from build123d import *

# Parameters (mm, degrees)
SKETCH1_R           = 2.1
BOSS_EXTRUDE1_DEPTH = 3
EXTRUDE_THIN1_DEPTH = 47
BOSS_EXTRUDE2_DEPTH = 3
SKETCH4_W           = 31
SKETCH4_H           = 51
CUT_EXTRUDE1_DEPTH  = 72.0791812
FILLET3_R           = 5
BOSS_EXTRUDE3_DEPTH = 30
FILLET1_R           = 5
CUT_EXTRUDE3_REACH  = 75.33
SKETCH10_R          = 0.5
SKETCH11_R          = 4.15
CUT_EXTRUDE4_DEPTH  = 1
FILLET2_R           = 5


with BuildPart() as part:
    # Sketch1 → Boss-Extrude1 (new body)
    with BuildSketch(Plane.XY):
        with BuildLine():
            Line((7.416198487, 5), (23.5, 5))
            Line((23.5, 5), (23.5, -25))
            Line((23.5, -25), (-23.5, -25))
            Line((-23.5, -25), (-23.5, 5))
            Line((-23.5, 5), (-7.416198487, 5))
            ThreePointArc((-7.416198487, 5), (0, 0), (7.416198487, 5))
        make_face()
        with Locations((-17.5, 0)):
            Circle(SKETCH1_R, mode=Mode.SUBTRACT)
        with Locations(Location((17.5, 0, 0), (0, 0, 180))):
            Circle(SKETCH1_R, mode=Mode.SUBTRACT)
    extrude(amount=BOSS_EXTRUDE1_DEPTH)

    # Sketch2 → Extrude-Thin1 (add)
    with BuildSketch(Plane.ZY.offset(23.5)):
        Polygon((0, -25), (-60, -25), (-60, 5), (-57, 5), (-57, -22), (0, -22), align=None)
    extrude(amount=-EXTRUDE_THIN1_DEPTH)

    # Sketch3 → Boss-Extrude2 (add)
    with BuildSketch(Plane.ZY.offset(23.5)):
        Polygon((-57, 5), (-57, -22), (0, -22), (0, 5), (-17.944444444, -12), (-39.055555556, -12), align=None)
    boss_extrude2 = extrude(amount=-BOSS_EXTRUDE2_DEPTH)

    # Mirror1: Boss-Extrude2 across plane
    add(boss_extrude2.mirror(Plane(origin=(0, 0, 0), x_dir=(0, 0, 1), z_dir=(1, 0, 0))))

    # Sketch4 → Cut-Extrude1 (cut, through all)
    with BuildSketch(Plane.XZ.offset(25)):
        with Locations((0, -28.5)):
            Rectangle(SKETCH4_W, SKETCH4_H)
    extrude(amount=-CUT_EXTRUDE1_DEPTH, mode=Mode.SUBTRACT)

    # Fillet3
    fillet3_edges = [part.edges().sort_by_distance(p)[0] for p in [
        (15.5, -23.5, -3),
        (15.5, -23.5, -54),
        (-15.5, -23.5, -54),
        (-15.5, -23.5, -3),
    ]]
    fillet(fillet3_edges, radius=FILLET3_R)

    # Sketch6 → Boss-Extrude3 (add)
    with BuildSketch(Plane(origin=(0, 5, 0), x_dir=(1, 0, 0), z_dir=(0, 1, 0))):
        Polygon((20.5, 57), (23.5, 57), (23.5, 60), (-23.5, 60), (-23.5, 57), (-20.5, 57), align=None)
    extrude(amount=BOSS_EXTRUDE3_DEPTH)

    # Fillet1
    fillet1_edges = [part.edges().sort_by_distance(p)[0] for p in [
        (-20.5, -22, -28.5),
        (20.5, -22, -28.5),
    ]]
    fillet(fillet1_edges, radius=FILLET1_R - 0.0001)  # a hair under: the kernel refuses the full size

    # Sketch10 → Cut-Extrude3 (cut, up to next)
    with BuildSketch(Plane.XY.offset(-57), mode=Mode.PRIVATE) as cut_extrude3_sk1:
        with Locations((0, 8)):
            Circle(SKETCH10_R)
    cut_extrude3_tool1 = extrude(cut_extrude3_sk1.sketch, amount=-CUT_EXTRUDE3_REACH, mode=Mode.PRIVATE) & part.part
    add(cut_extrude3_tool1.solids().sort_by_distance((0, 8, -57))[0], mode=Mode.SUBTRACT)

    # Sketch11 → Cut-Extrude4 (cut)
    with BuildSketch(Plane(origin=(0, 0, -60), x_dir=(-1, 0, 0), z_dir=(0, 0, -1))):
        with Locations((-18.5, 30)):
            Circle(SKETCH11_R)
        with Locations((18.5, 30)):
            Circle(SKETCH11_R)
        with Locations((-18.5, -20)):
            Circle(SKETCH11_R)
        with Locations((18.5, -20)):
            Circle(SKETCH11_R)
    extrude(amount=-CUT_EXTRUDE4_DEPTH, mode=Mode.SUBTRACT)

    # Fillet2
    fillet2_edges = [part.edges().sort_by_distance(p)[0] for p in [
        (23.5, 35, -58.5),
        (-23.5, 35, -58.5),
    ]]
    fillet(fillet2_edges, radius=FILLET2_R)


solid = part.part
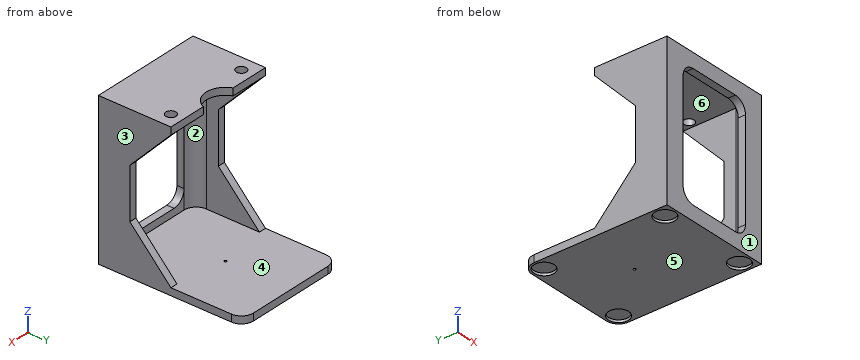
Design review of the part built by this model. Coordinates are the model's own, in mm. Face numbers are marked on the shaded views. A direction names the side the tool comes from. Round coordinates to 2 decimals unless told otherwise and drop trailing zeros. Loops run counter-clockwise (first coordinate to the right, second up) from the corner with the lowest first, then second, coordinate; pieces in that order, holes last. Notation, with made-up numbers: (-18.75, 69) - (3.25, 69) arc R20 ccw to (3.25, 75) - close; hole circle Ø10 at (30.5, -32.75). An arc over 180 degrees is marked (long way). One line per question, with ' | ' between items.
1. We need section D-D, the plane x = 1.5. State the section outline as (y, z) points.
Results are:
outline: (-25, -60) - (35, -60) - (35, -57) - (-22, -57) - (-22, -54) - (-25, -54) - close; (-25, -3) - (-22, -3) - (-22, 0) - (0.14, 0) - (0.14, 3) - (-25, 3) - close
2. Draft analysis for pull direction X (two halves, no side actions). For the marked faces 3, 4, 5 and 6, state which applies: released by +X, released by -X, zero draft, split by the parting line, or undercut.
Results are:
face 3: released by +X | face 4: undercut | face 5: zero draft | face 6: undercut
3. We need section A-A, the plane x = 17.5. State the section outline as (y, z) points, and give its area (3 significant figures).
Results are:
outline: (-25, -60) - (-24.03, -60) - (-24.03, -59) - (-15.97, -59) - (-15.97, -60) - (25.97, -60) - (25.97, -59) - (34.03, -59) - (34.03, -60) - (35, -60) - (35, -57) - (-21.58, -57) - (-21.58, 0) - (-2.1, 0) - (-2.1, 3) - (-25, 3) - close; (2.1, 0) - (5, 0) - (5, 3) - (2.1, 3) - close | area: 436 mm²
4. For the marked faces 1 and 2, list the 3-axis set-ups (+Z, -Z, +X, -X, +Y, -Y) from which the entire face can be reached by the end or side of a thin tool; tool diameter is ignored.
Results are:
face 1: +Z, -Z, +X, -X, -Y | face 2: +Y
5. For L1, parallel to Y at x = 18.5, z = -59.3; L2, parallel to Y at x = 17.5, z = 0.95; L3, parallel to Y at x = 0, z = -58.1, list the stretches that pass through material, from the lowest coordinate up. Write a range as [from, to].
Results are:
L1: y = [-25, -24.15], [-15.85, 25.85], [34.15, 35] | L2: y = [-25, -2.1], [2.1, 5] | L3: y = [-25, 7.5], [8.5, 35]
6. Clearance check with flat-ended pins moving along their axes: P1, Ø2.5, axis at x = -17, z = 1, coming from the +Y side; P2, Ø6.5, axis at x = 19.5, y = -19.5, coming from the -Z side; P3, Ø2.5, axis at x = 22, z = -29.5, coming from the +Y side; P4, Ø9.5, axis at x = 18.5, y = 30, coming from the +Z side. State where each tip first meets the part, or that it passes through.
Results are:
P1: stops at y = 5 | P2: stops at z = -60 | P3: stops at y = -12 | P4: stops at z = -57
7. We need section B-B, the plane y = -14.5. State the section outline as (x, z) points.
Results are:
outline: (-23.5, -60) - (23.5, -60) - (23.5, 3) - (-23.5, 3) - close; hole (-20.5, -57) - (20.5, -57) - (20.5, 0) - (-20.5, 0) - close
